Work out the finished part from the listing and answer in its coordinate system (mm). Give positions to 0.01 mm unless a question says otherwise; leave off trailing zeros. Loops run counter-clockwise (first coordinate to the right, second up) from the corner with the lowest first, then second, coordinate; pieces in that order, holes last. Notation, with made-up numbers: M 35,63 L 94,63 A25 ccw 94,99 Z; hole C 76.5,59 d8. An arc over 180 degrees is marked long. Write item = value, one per line. Start each with the question number.
1. Flat-ended cylindrical pins translate along their axes: pin 1 Ø4 at (x, z) = (0, 42.5) entering from -Y; pin 2 Ø4 at (x, z) = (-3.5, 44.5) entering from -Y; pin 3 Ø6 at (x, z) = (-0.5, 22) entering from +Y. Find the tip coordinate at first contact, or state that the pin passes through.
2. Consider L1, parallel to Y at x = 0, z = 4.75; L2, parallel to Y at x = 0, z = 59.4; L3, parallel to Z at x = 1.5, y = 1. Determine where each line is inside the solid, lowest interval first. Write a range as [from, to].
3. Section A-A on y = 0 is taken. Determine the outline of the cut face in (x, z).
```python
from build123d import *

# Parameters (mm, degrees)
SKETCH1_W           = 15
SKETCH1_H           = 15
BOSS_EXTRUDE1_DEPTH = 60
BOSS_EXTRUDE1_TAPER = 2
SKETCH2_R           = 1.5
CUT_EXTRUDE1_DEPTH  = 10
SKETCH3_R           = 2.75
CUT_EXTRUDE2_DEPTH  = 2
FILLET1_R           = 1.5


with BuildPart() as part:
    # Sketch1 → Boss-Extrude1 (new body)
    with BuildSketch(Plane.XY):
        Rectangle(SKETCH1_W, SKETCH1_H)
    extrude(amount=BOSS_EXTRUDE1_DEPTH, taper=BOSS_EXTRUDE1_TAPER)

    # Sketch2 → Cut-Extrude1 (cut)
    with BuildSketch(Plane(origin=(0, 0, 0), x_dir=(-1, 0, 0), z_dir=(0, 0, -1))):
        Circle(SKETCH2_R)
    extrude(amount=-CUT_EXTRUDE1_DEPTH, mode=Mode.SUBTRACT)

    # Sketch3 → Cut-Extrude2 (cut)
    with BuildSketch(Plane.XY.offset(60)):
        Circle(SKETCH3_R)
    extrude(amount=-CUT_EXTRUDE2_DEPTH, mode=Mode.SUBTRACT)

    # Fillet1
    fillet1_edges = [part.edges().sort_by_distance(p)[0] for p in [
        (-5.40475383, 0, 60),
        (0, -5.40475383, 60),
        (5.40475383, 0, 60),
        (6.452376915, -6.452376915, 30),
        (-6.452376915, -6.452376915, 30),
        (-6.452376453, 6.452376453, 30.000013228),
        (6.452376915, 6.452376915, 30),
        (0, 5.40475383, 60),
    ]]
    fillet(fillet1_edges, radius=FILLET1_R)


solid = part.part
```
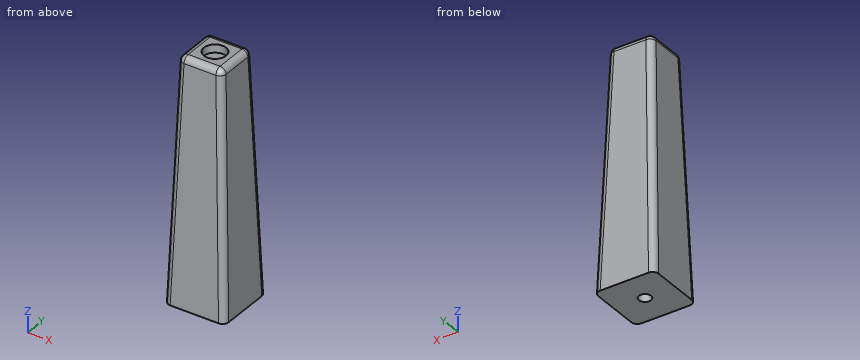
Verdict:
q1.pin_1 = -6.09
q1.pin_2 = -6.02
q1.pin_3 = 6.84
q2.L1 = [-7.33, -1.5], [1.5, 7.33]
q2.L2 = [-5.16, -2.75], [2.75, 5.16]
q2.L3 = [0, 58]
q3.outline = M -7.5,0 L -1.5,0 L -1.5,10 L 1.5,10 L 1.5,0 L 7.5,0 L 5.46,58.55 A1.5 ccw 3.96,60 L 2.75,60 L 2.75,58 L -2.75,58 L -2.75,60 L -3.96,60 A1.5 ccw -5.46,58.55 Z
